Input: part model. Units: mm. Frame: model coordinates. A direction names the side the tool comes from. Coordinates: 2 decimals unless noted, no trailing zeros. Loops run counter-clockwise (first coordinate to the right, second up) from the corner with the lowest first, then second, coordinate; pieces in that order, holes last. Notation, with made-up numbers: (-7.75, 9) -> (11.25, 9) arc R18 ccw to (11.25, 23) -> close; hole circle Ø11 at (-17, 55.25). An arc over 180 degrees is marked (long way). Put each result on its own line as item: value. Start each with the question number.
1) Contact query for flat-ended pins moving along their axis: P1, Ø3, axis at y = 49.2, z = 88.11, coming from the -X side; P2, Ø1.5, axis at x = -40.5, y = 102.5, coming from the -Z side; P3, Ø8, axis at x = -20, y = -66.5, coming from the +Z side. Output: stop coordinate, or through.
2) Cut plane C-C (y = 57.5). Return the cut outline in (x, z), plus the area to 3 significant figures.
3) Cut plane A-A (z = 76.2). State how many separate pieces and enclosed holes the cut face has, plus the area to 3 significant figures.
4) Pull-direction query (Z, two-part tool) for faces 4 (the flat face through (-1, 2, 0)), 5 (the cylindrical face through (0.533, 28.994, 85.716)), 6 (the flat face through (38.1, 33, 85)), 7 (the flat face through (-1, 29, 152.4)); classes: pulls with the +Z half, pulls with the -Z half, needs draft (parallel to the pull), parting line crosses it, or undercut.
5) Material intervals for L1, parallel to Y at x = -1, z = 63 (3 decimals); L2, parallel to Y at x = -20.5, z = 76.2 (3 decimals); L3, parallel to X at y = -26, z = 134, sorted ascending.
6) Set-up query: faces 1 (the cylindrical face through (37.622, 3.52, 12.522)), 2 (the cylindrical face through (11.968, -69.756, 62.323)), 3 (the cylindrical face through (-3.09, 39.81, 146.14)). Return all of +Z, -Z, +X, -X, +Y, -Y with unobstructed straight access to the full face (end or side cutting, diameter ignored); none if empty.
from build123d import *

# Parameters (mm, degrees)
SKETCH1_W                       = 101.6
SKETCH1_H                       = 247.65
BOSS_EXTRUDE1_DEPTH             = 152.4
SKETCH2_R                       = 15.08125
SKETCH2_R_2                     = 9.525
CUT_EXTRUDE1_DEPTH              = 203.827588422
SKETCH33_R                      = 2.5796875
CUT_EXTRUDE33_DEPTH             = 25.4
SKETCH53_R                      = 31.75
CUT_EXTRUDE37_DEPTH             = 24.13
SKETCH54_R                      = 19.05
CUT_EXTRUDE38_DEPTH             = 38.1
SKETCH4_R                       = 19.05
CUT_EXTRUDE40_DEPTH             = 12.7
SKETCH56_R                      = 14.2494
CUT_EXTRUDE42_DEPTH             = 12.7
CUT_EXTRUDE43_START             = -12.7
SKETCH57_R                      = 14.2494
CUT_EXTRUDE43_DEPTH             = 12.7
SKETCH58_R                      = 25.4
CUT_EXTRUDE44_DEPTH             = 50.8
CUT_EXTRUDE45_DEPTH             = 127
FILLET2_R                       = 0.00254
CUT_EXTRUDE46_START             = -12.7
SKETCH60_R                      = 19.05
CUT_EXTRUDE46_DEPTH             = 12.7
SKETCH61_R                      = 9.525
CUT_EXTRUDE47_DEPTH             = 222.090367554
F_10_32_TAPPED_HOLE1_D          = 4.0386
F_10_32_TAPPED_HOLE1_DEPTH      = 25.4
F_10_32_TAPPED_HOLE1_TIP        = 1.213317848
F_10_32_TAPPED_HOLE2_AT_2_COUNT = 2
F_10_32_TAPPED_HOLE2_AT_2_PITCH = 23.8125
F_10_32_TAPPED_HOLE2_AT_3_COUNT = 2
F_10_32_TAPPED_HOLE2_AT_3_PITCH = 23.8125
F_10_32_TAPPED_HOLE2_AT_4_COUNT = 2
F_10_32_TAPPED_HOLE2_AT_4_PITCH = 41.244459855
F_10_32_TAPPED_HOLE2_AT_5_COUNT = 2
F_10_32_TAPPED_HOLE2_AT_5_PITCH = 47.625
F_10_32_TAPPED_HOLE2_AT_6_COUNT = 2
F_10_32_TAPPED_HOLE2_AT_6_PITCH = 41.244459855
F_1_4_20_TAPPED_HOLE1_D         = 5.1054
F_1_4_20_TAPPED_HOLE1_DEPTH     = 19.05
F_1_4_20_TAPPED_HOLE1_TIP       = 1.533816902


with BuildPart() as part:
    # Sketch1 → Boss-Extrude1 (new body)
    with BuildSketch(Plane.XY):
        Rectangle(SKETCH1_W, SKETCH1_H)
    extrude(amount=BOSS_EXTRUDE1_DEPTH)

    # Sketch2 → Cut-Extrude1 (cut, through all)
    with BuildSketch(Plane(origin=(0, 0, 0), x_dir=(-1, 0, 0), z_dir=(0, 0, -1))):
        with Locations((0, -60.579)):
            Circle(SKETCH2_R)
        with Locations((0, 53.721)):
            Circle(SKETCH2_R_2)
    extrude(amount=-CUT_EXTRUDE1_DEPTH, mode=Mode.SUBTRACT)

    # Sketch33 → Cut-Extrude33 (cut)
    with BuildSketch(Plane(origin=(0, 0, 0), x_dir=(-1, 0, 0), z_dir=(0, 0, -1))):
        with Locations((-40.005, 102.9335)):
            Circle(SKETCH33_R)
        with Locations((40.005, 102.9335)):
            Circle(SKETCH33_R)
        with Locations((40.005, 4.5085)):
            Circle(SKETCH33_R)
        with Locations((-40.005, 4.5085)):
            Circle(SKETCH33_R)
    extrude(amount=-CUT_EXTRUDE33_DEPTH, mode=Mode.SUBTRACT)

    # Sketch53 → Cut-Extrude37 (cut)
    with BuildSketch(Plane(origin=(0, 0, 0), x_dir=(-1, 0, 0), z_dir=(0, 0, -1))):
        with Locations((0, -60.579)):
            Circle(SKETCH53_R)
    extrude(amount=-CUT_EXTRUDE37_DEPTH, mode=Mode.SUBTRACT)

    # Sketch54 → Cut-Extrude38 (cut)
    with BuildSketch(Plane(origin=(0, 0, 0), x_dir=(-1, 0, 0), z_dir=(0, 0, -1))):
        with Locations((0, 53.721)):
            Circle(SKETCH54_R)
    extrude(amount=-CUT_EXTRUDE38_DEPTH, mode=Mode.SUBTRACT)

    # Sketch4 → Cut-Extrude40 (cut)
    with BuildSketch(Plane(origin=(50.8, 0, 0), x_dir=(0, 0, -1), z_dir=(1, 0, 0))):
        with Locations((-76.2, 28.575)):
            Circle(SKETCH4_R)
    extrude(amount=-CUT_EXTRUDE40_DEPTH, mode=Mode.SUBTRACT)

    # Sketch56 → Cut-Extrude42 (cut)
    with BuildSketch(Plane.XY.offset(152.4)):
        with Locations((0, 53.721)):
            Circle(SKETCH56_R)
    extrude(amount=-CUT_EXTRUDE42_DEPTH, mode=Mode.SUBTRACT)

    # Sketch57 → Cut-Extrude43 (cut)
    with BuildSketch(Plane(origin=(0, 0, 38.1), x_dir=(-1, 0, 0), z_dir=(0, 0, -1)).offset(CUT_EXTRUDE43_START)):
        with Locations(Location((0, 53.721, 0), (0, 0, 180))):
            Circle(SKETCH57_R)
    extrude(amount=CUT_EXTRUDE43_DEPTH, mode=Mode.SUBTRACT)

    # Sketch58 → Cut-Extrude44 (cut)
    with BuildSketch(Plane.XY.offset(152.4)):
        with Locations((0, -60.579)):
            Circle(SKETCH58_R)
    extrude(amount=-CUT_EXTRUDE44_DEPTH, mode=Mode.SUBTRACT)

    # Sketch59 → Cut-Extrude45 (cut)
    with BuildSketch(Plane.XY.offset(152.4)):
        with BuildLine():
            ThreePointArc((-17.734642857, -13.34047826), (20.0025, -4.0894), (-17.734642857, 5.16167826))
            ThreePointArc((-17.734642857, 5.16167826), (-29.5275, -4.0894), (-17.734642857, -13.34047826))
        make_face()
    extrude(amount=-CUT_EXTRUDE45_DEPTH, mode=Mode.SUBTRACT)

    # Fillet2
    fillet2_edges = [part.edges().sort_by_distance(p)[0] for p in [
        (50.8, -123.825, 76.2),
        (-50.8, -123.825, 76.2),
        (-50.8, 123.825, 76.2),
        (50.8, 123.825, 76.2),
    ]]
    fillet(fillet2_edges, radius=FILLET2_R)

    # Sketch60 → Cut-Extrude46 (cut)
    with BuildSketch(Plane.ZY.offset(50.8).offset(CUT_EXTRUDE46_START)):
        with Locations(Location((76.2, 28.575, 0), (0, 0, 180))):
            Circle(SKETCH60_R)
    extrude(amount=CUT_EXTRUDE46_DEPTH, mode=Mode.SUBTRACT)

    # Sketch61 → Cut-Extrude47 (cut, through all)
    with BuildSketch(Plane(origin=(50.8, 0, 0), x_dir=(0, 0, -1), z_dir=(1, 0, 0))):
        with Locations((-76.2, 28.575)):
            Circle(SKETCH61_R)
    extrude(amount=-CUT_EXTRUDE47_DEPTH, mode=Mode.SUBTRACT)

    # #10-32 Tapped Hole1
    with Locations(Plane.XY.offset(152.4)):
        with Locations((-22.225, 18.1356), (22.225, 18.1356), (22.225, -26.3144), (-22.225, -26.3144)):
            Hole(F_10_32_TAPPED_HOLE1_D / 2, depth=F_10_32_TAPPED_HOLE1_DEPTH)
            with Locations((0, 0, -(F_10_32_TAPPED_HOLE1_DEPTH + F_10_32_TAPPED_HOLE1_TIP / 2))):  # 118° drill point
                Cone(0, F_10_32_TAPPED_HOLE1_D / 2, F_10_32_TAPPED_HOLE1_TIP, mode=Mode.SUBTRACT)

    # Sketch66 → #10-32 Tapped Hole2 (revolve, cut)
    with BuildSketch(Plane(origin=(-50.8, 7.952770072, 64.29375), x_dir=(0, 0, 1), z_dir=(0, 1, 0))):
        Polygon((0, 0), (0, 26.613317848), (2.0193, 25.4), (2.0193, 0), align=None)
    f_10_32_tapped_hole2 = revolve(axis=Axis((-57.15, 7.952770072, 64.29375), (1, 0, 0)), mode=Mode.SUBTRACT)

    # #10-32 Tapped Hole2 at 2: #10-32 Tapped Hole2 ×2
    with Locations(*[Vector(0, 0.8660254037844412, -0.4999999999999957) * (i * F_10_32_TAPPED_HOLE2_AT_2_PITCH) for i in range(1, F_10_32_TAPPED_HOLE2_AT_2_COUNT)]):
        add(f_10_32_tapped_hole2, mode=Mode.SUBTRACT)

    # #10-32 Tapped Hole2 at 3: #10-32 Tapped Hole2 ×2
    with Locations(*[(0, 0, i * F_10_32_TAPPED_HOLE2_AT_3_PITCH) for i in range(1, F_10_32_TAPPED_HOLE2_AT_3_COUNT)]):
        add(f_10_32_tapped_hole2, mode=Mode.SUBTRACT)

    # #10-32 Tapped Hole2 at 4: #10-32 Tapped Hole2 ×2
    with Locations(*[Vector(0, 0.49999999999999195, 0.8660254037844434) * (i * F_10_32_TAPPED_HOLE2_AT_4_PITCH) for i in range(1, F_10_32_TAPPED_HOLE2_AT_4_COUNT)]):
        add(f_10_32_tapped_hole2, mode=Mode.SUBTRACT)

    # #10-32 Tapped Hole2 at 5: #10-32 Tapped Hole2 ×2
    with Locations(*[Vector(0, 0.8660254037844348, 0.5000000000000068) * (i * F_10_32_TAPPED_HOLE2_AT_5_PITCH) for i in range(1, F_10_32_TAPPED_HOLE2_AT_5_COUNT)]):
        add(f_10_32_tapped_hole2, mode=Mode.SUBTRACT)

    # #10-32 Tapped Hole2 at 6: #10-32 Tapped Hole2 ×2
    with Locations(*[(0, i * F_10_32_TAPPED_HOLE2_AT_6_PITCH, 0) for i in range(1, F_10_32_TAPPED_HOLE2_AT_6_COUNT)]):
        add(f_10_32_tapped_hole2, mode=Mode.SUBTRACT)

    # Mirror1: #10-32 Tapped Hole2 across plane
    add(f_10_32_tapped_hole2.mirror(Plane(origin=(0, 0, 0), x_dir=(0, 0, 1), z_dir=(1, 0, 0))), mode=Mode.SUBTRACT)

    # Mirror1 copy 1 sketch → Mirror1 copy 1 (revolve, cut)
    with BuildSketch(Plane(origin=(50.8, 28.575, 52.3875), x_dir=(0, 0, 1), z_dir=(0, 1, 0))):
        Polygon((0, 0), (0, -26.613317848), (2.0193, -25.4), (2.0193, 0), align=None)
    revolve(axis=Axis((57.15, 28.575, 52.3875), (1, 0, 0)), mode=Mode.SUBTRACT)

    # Mirror1 copy 2 sketch → Mirror1 copy 2 (revolve, cut)
    with BuildSketch(Plane(origin=(50.8, 7.952770072, 88.10625), x_dir=(0, 0, 1), z_dir=(0, 1, 0))):
        Polygon((0, 0), (0, -26.613317848), (2.0193, -25.4), (2.0193, 0), align=None)
    revolve(axis=Axis((57.15, 7.952770072, 88.10625), (1, 0, 0)), mode=Mode.SUBTRACT)

    # Mirror1 copy 3 sketch → Mirror1 copy 3 (revolve, cut)
    with BuildSketch(Plane(origin=(50.8, 28.575, 100.0125), x_dir=(0, 0, 1), z_dir=(0, 1, 0))):
        Polygon((0, 0), (0, -26.613317848), (2.0193, -25.4), (2.0193, 0), align=None)
    revolve(axis=Axis((57.15, 28.575, 100.0125), (1, 0, 0)), mode=Mode.SUBTRACT)

    # Mirror1 copy 4 sketch → Mirror1 copy 4 (revolve, cut)
    with BuildSketch(Plane(origin=(50.8, 49.197229928, 88.10625), x_dir=(0, 0, 1), z_dir=(0, 1, 0))):
        Polygon((0, 0), (0, -26.613317848), (2.0193, -25.4), (2.0193, 0), align=None)
    revolve(axis=Axis((57.15, 49.197229928, 88.10625), (1, 0, 0)), mode=Mode.SUBTRACT)

    # Mirror1 copy 5 sketch → Mirror1 copy 5 (revolve, cut)
    with BuildSketch(Plane(origin=(50.8, 49.197229928, 64.29375), x_dir=(0, 0, 1), z_dir=(0, 1, 0))):
        Polygon((0, 0), (0, -26.613317848), (2.0193, -25.4), (2.0193, 0), align=None)
    revolve(axis=Axis((57.15, 49.197229928, 64.29375), (1, 0, 0)), mode=Mode.SUBTRACT)

    # 1/4-20 Tapped Hole1
    with Locations(Plane.XY.offset(152.4)):
        with Locations((-44.45, 19.05), (-44.45, -6.35)):
            Hole(F_1_4_20_TAPPED_HOLE1_D / 2, depth=F_1_4_20_TAPPED_HOLE1_DEPTH)
            with Locations((0, 0, -(F_1_4_20_TAPPED_HOLE1_DEPTH + F_1_4_20_TAPPED_HOLE1_TIP / 2))):  # 118° drill point
                Cone(0, F_1_4_20_TAPPED_HOLE1_D / 2, F_1_4_20_TAPPED_HOLE1_TIP, mode=Mode.SUBTRACT)


solid = part.part
Results found:
1. P1: stops at x = -25.09
1. P2: stops at z = 25.4
1. P3: stops at z = 101.6
2. outline: (-50.8, 0) -> (-18.67, 0) -> (-18.67, 38.1) -> (-13.74, 38.1) -> (-13.74, 50.8) -> (-8.74, 50.8) -> (-8.74, 139.7) -> (-13.74, 139.7) -> (-13.74, 152.4) -> (-50.8, 152.4) -> close; (8.74, 50.8) -> (13.74, 50.8) -> (13.74, 38.1) -> (18.67, 38.1) -> (18.67, 0) -> (50.8, 0) -> (50.8, 152.4) -> (13.74, 152.4) -> (13.74, 139.7) -> (8.74, 139.7) -> close
2. area: 11,800 mm2
3. separate pieces: 2
3. enclosed holes: 3
3. area: 20,300 mm2
4. face 4: pulls with the -Z half
4. face 5: undercut
4. face 6: undercut
4. face 7: pulls with the +Z half
5. L1: y = -123.825 to -75.627, -45.531 to -24.067, 15.888 to 44.249, 63.193 to 123.825
5. L2: y = -123.825 to -13.601, 5.423 to 19.05, 38.1 to 123.825
5. L3: x = -50.8 to -24.22, -20.23 to 20.23, 24.22 to 50.8
6. face 1: -Z
6. face 2: +Z, -Z
6. face 3: +Z
